Verification items for the finished model (mm, model axes). A direction names the side the tool comes from. Coordinates: 2 decimals unless noted, no trailing zeros. Write each loop counter-clockwise with the first axis right and the second up, starting at its lowest first coordinate (ties: lowest second). Pieces come first, ordered by that corner, then holes. Notation, with made-up numbers: (75, 52.5) -> (82, 52.5) arc R20 ccw to (82, 82.5) -> close; hole circle Ø7 at (16.25, 26). An arc over 180 degrees is marked (long way). Answer in a Markdown table with one row per item.
```python
from build123d import *

# Parameters (mm, degrees)
SKETCH1_R           = 3.625
BOSS_EXTRUDE1_DEPTH = 6.82
CHAMFER1_SIZE       = 0.5
SKETCH2_W           = 3.2
SKETCH2_H           = 3.2
CUT_EXTRUDE1_DEPTH  = 2.93


with BuildPart() as part:
    # Sketch1 → Boss-Extrude1 (new body)
    with BuildSketch(Plane(origin=(0, 0, 0), x_dir=(1, 0, 0), z_dir=(0, 1, 0))):
        Circle(SKETCH1_R)
    extrude(amount=BOSS_EXTRUDE1_DEPTH)

    # Chamfer1
    chamfer1_edges = [part.edges().sort_by_distance(p)[0] for p in [
        (-3.625, 6.82, 0),
    ]]
    chamfer(chamfer1_edges, length=CHAMFER1_SIZE)

    # Sketch2 → Cut-Extrude1 (cut)
    with BuildSketch(Plane.XZ):
        Rectangle(SKETCH2_W, SKETCH2_H)
    extrude(amount=-CUT_EXTRUDE1_DEPTH, mode=Mode.SUBTRACT)


solid = part.part
```
1. Release check for a two-part mould opening along Z. For faces 1 (the face through (-2, 0, 0)), 2 (the face through (0, 1, 1.6)), 3 (the face through (1.7, 3.1, 3.2)), 4 (the face through (-1.6, 1, 0)) record: released by +Z, released by -Z, zero draft, split by the parting line, or undercut.
Findings below:
| item | result |
|---|---|
| face 1 | zero draft |
| face 2 | undercut |
| face 3 | split by the parting line |
| face 4 | undercut |
2. Sectioned sample at A-A, the plane y = 1.5. Record the cut outline in (x, z) (3 decimals), and give its area (3 significant figures).
Findings below:
| item | result |
|---|---|
| outline | circle Ø7.25 at (0, 0); hole (-1.6, -1.6) -> (1.6, -1.6) -> (1.6, 1.6) -> (-1.6, 1.6) -> close |
| area | 31.0 mm² |
3. Sectioned sample at C-C, the plane z = 0. Record the cut outline in (x, y) (3 decimals).
Findings below:
| item | result |
|---|---|
| outline | (-3.625, 0) -> (-1.6, 0) -> (-1.6, 2.93) -> (1.6, 2.93) -> (1.6, 0) -> (3.625, 0) -> (3.625, 6.32) -> (3.125, 6.82) -> (-3.125, 6.82) -> (-3.625, 6.32) -> close |
4. Access from +Z, -Z, +X, -X, +Y, -Y to the whole of each face (thin tool, end or side, straight path). Record for faces 5 (the face through (0, 6.82, 0)), 6 (the face through (0, 2.93, 0)).
Findings below:
| item | result |
|---|---|
| face 5 | +Z, -Z, +X, -X, +Y |
| face 6 | -Y |
5. Sectioned sample at D-D, the plane y = 4.25. Record the cut outline in (x, z) (3 decimals), and give its area (3 significant figures).
Findings below:
| item | result |
|---|---|
| outline | circle Ø7.25 at (0, 0) |
| area | 41.3 mm² |
6. Material ranges on probe 1 along Z at (x, y) = (0, 1.25) (3 decimals); probe 2 along Y at (x, z) = (0, -0.25); probe 3 along Z at (x, y) = (1.5, 1), recorded low to high. Write a range as from..to.
Findings below:
| item | result |
|---|---|
| probe 1 | z = -3.625..-1.6, 1.6..3.625 |
| probe 2 | y = 2.93..6.82 |
| probe 3 | z = -3.3..-1.6, 1.6..3.3 |
7. Sectioned sample at B-B, the plane x = 0. Record the cut outline in (y, z) (3 decimals), and give its area (3 significant figures).
Findings below:
| item | result |
|---|---|
| outline | (0, -3.625) -> (6.32, -3.625) -> (6.82, -3.125) -> (6.82, 3.125) -> (6.32, 3.625) -> (0, 3.625) -> (0, 1.6) -> (2.93, 1.6) -> (2.93, -1.6) -> (0, -1.6) -> close |
| area | 39.8 mm² |
